Could you check a few things on this model? Use its own coordinates, in mm. Face numbers are marked on the shaded views. A direction names the side the tool comes from. Coordinates: 2 decimals unless noted, no trailing zeros. Loops run counter-clockwise (first coordinate to the right, second up) from the corner with the lowest first, then second, coordinate; pieces in that order, holes last.
1) Imagine slicing it at C-C on y = 6.35. Please give me the cut outline in (x, z).
2) Imagine slicing it at D-D on y = 8.5. Please give me the cut outline in (x, z), plus the area to 3 significant figures.
3) For the marked faces 1 and 2, which set-ups out of +Z, -Z, +X, -X, +Y, -Y let a thin tool reach every point of the face, with its end or its side?
4) Will these pins go through, and if not, where does the flat tip stop? P1, Ø3.5, axis at x = 7.82, y = 6.35, coming from the +Z side; P2, Ø2, axis at x = 0.5, y = 10.5, coming from the +Z side; P3, Ø10, axis at x = 0.5, z = -4.5, coming from the +Y side; P4, Ø3, axis at x = 8.5, y = 7.5, coming from the -Z side.
5) Imagine slicing it at A-A on x = 0. Please give me the cut outline in (y, z), plus the area to 3 significant figures.
6) Thinking about a two-plate mould opening in Z: for the marked faces 3, 4, 5 and 6, which applies, released by +Z, released by -Z, zero draft, split by the parting line, or undercut?
7) If I drill on line 1 along X through (y, z) = (7.25, -13); line 2 along Y through (x, z) = (-7.75, -13.5); line 3 along Z through (x, y) = (3, 7), over which ranges is the centre line in solid material (lowest first)?
8) Imagine slicing it at B-B on z = -2. Please give me the cut outline in (x, y).
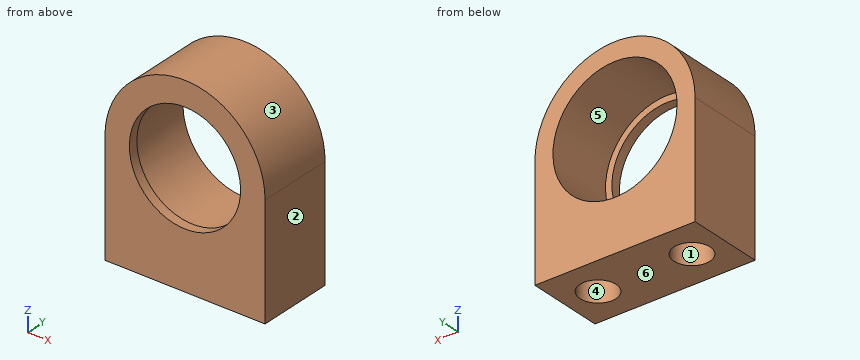
```python
from build123d import *

# Parameters (mm, degrees)
SKETCH1_R           = 9.25
BOSS_EXTRUDE1_DEPTH = 12.7
SKETCH2_R           = 10.31875
CUT_EXTRUDE1_DEPTH  = 11.1125
SKETCH3_R           = 3
CUT_EXTRUDE2_DEPTH  = 7.5
BOSS_EXTRUDE2_START = 1
SKETCH4_W           = 26.6375
SKETCH4_H           = 12.7
SKETCH4_R           = 3
BOSS_EXTRUDE2_DEPTH = 1


with BuildPart() as part:
    # Sketch1 → Boss-Extrude1 (new body)
    with BuildSketch(Plane(origin=(0, 0, 0), x_dir=(1, 0, 0), z_dir=(0, 1, 0))):
        with BuildLine():
            Line((-13.31875, 0), (-13.31875, 13.31875))
            Line((-13.31875, 13.31875), (-13.31875, 17.81875))
            Line((-13.31875, 17.81875), (13.31875, 17.81875))
            Line((13.31875, 17.81875), (13.31875, 13.31875))
            Line((13.31875, 13.31875), (13.31875, 0))
            ThreePointArc((13.31875, 0), (0, -13.31875), (-13.31875, 0))
        make_face()
        with Locations(Location((0, 0, 0), (0, 0, 270))):
            Circle(SKETCH1_R, mode=Mode.SUBTRACT)
    extrude(amount=BOSS_EXTRUDE1_DEPTH)

    # Sketch2 → Cut-Extrude1 (cut)
    with BuildSketch(Plane(origin=(0, 12.7, 0), x_dir=(1, 0, 0), z_dir=(0, 1, 0))):
        with Locations(Location((0, 0, 0), (0, 0, 270))):
            Circle(SKETCH2_R)
    extrude(amount=-CUT_EXTRUDE1_DEPTH, mode=Mode.SUBTRACT)

    # Sketch3 → Cut-Extrude2 (cut)
    with BuildSketch(Plane(origin=(0, 0, -17.81875), x_dir=(-1, 0, 0), z_dir=(0, 0, -1))):
        with Locations((-7.81875, 6.35)):
            Circle(SKETCH3_R)
        with Locations((7.81875, 6.35)):
            Circle(SKETCH3_R)
    extrude(amount=-CUT_EXTRUDE2_DEPTH, mode=Mode.SUBTRACT)

    # Sketch4 → Boss-Extrude2 (add)
    with BuildSketch(Plane(origin=(0, 0, -17.81875), x_dir=(-1, 0, 0), z_dir=(0, 0, -1)).offset(BOSS_EXTRUDE2_START)):
        with Locations((0, 6.35)):
            Rectangle(SKETCH4_W, SKETCH4_H)
        with Locations((-7.81875, 6.35)):
            Circle(SKETCH4_R, mode=Mode.SUBTRACT)
        with Locations((7.81875, 6.35)):
            Circle(SKETCH4_R, mode=Mode.SUBTRACT)
    extrude(amount=-BOSS_EXTRUDE2_DEPTH)


solid = part.part
```
Filled in:
1. outline: (-13.32, -18.82) - (-10.82, -18.82) - (-10.82, -10.32) - (-4.82, -10.32) - (-4.82, -18.82) - (4.82, -18.82) - (4.82, -10.32) - (10.82, -10.32) - (10.82, -18.82) - (13.32, -18.82) - (13.32, 0) arc R13.32 ccw to (-13.32, 0) - close; hole circle Ø20.64 at (0, 0)
2. outline: (-13.32, -18.82) - (-9.91, -18.82) - (-9.91, -10.32) - (-5.73, -10.32) - (-5.73, -18.82) - (5.73, -18.82) - (5.73, -10.32) - (9.91, -10.32) - (9.91, -18.82) - (13.32, -18.82) - (13.32, 0) arc R13.32 ccw to (-13.32, 0) - close; hole circle Ø20.64 at (0, 0)
2. area: 374 mm2
3. face 1: -Z
3. face 2: +Z, -Z, +X, +Y, -Y
4. P1: stops at z = 11.86
4. P2: stops at z = 13.32
4. P3: stops at y = 1.59
4. P4: stops at z = -10.32
5. outline: (0, -18.82) - (12.7, -18.82) - (12.7, -10.32) - (1.59, -10.32) - (1.59, -9.25) - (0, -9.25) - close; (0, 9.25) - (1.59, 9.25) - (1.59, 10.32) - (12.7, 10.32) - (12.7, 13.32) - (0, 13.32) - close
5. area: 149 mm2
6. face 3: released by +Z
6. face 4: zero draft
6. face 5: undercut
6. face 6: released by -Z
7. line 1: x = -13.32 to -10.68, -4.96 to 4.96, 10.68 to 13.32
7. line 2: y = 0 to 3.35, 9.35 to 12.7
7. line 3: z = -18.82 to -9.87, 9.87 to 12.98
8. outline: (-13.32, 0) - (-9.03, 0) - (-9.03, 1.59) - (-10.12, 1.59) - (-10.12, 12.7) - (-13.32, 12.7) - close; (9.03, 0) - (13.32, 0) - (13.32, 12.7) - (10.12, 12.7) - (10.12, 1.59) - (9.03, 1.59) - close
